from build123d import *

# Parameters (mm, degrees)
SKETCH011_W     = 266
SKETCH011_H     = 55
PAD008_DEPTH    = 4
SKETCH021_W     = 40
SKETCH021_H     = 30
POCKET004_DEPTH = 4.001
SKETCH037_R     = 3.3
HOLE002_DEPTH   = 25


with BuildPart() as part:
    # Sketch011 (on DatumPlane) → Pad008 (new body)
    with BuildSketch(Plane(origin=(0, -83, -4), x_dir=(-1, 0, 0), z_dir=(0, 1, 0))):
        with Locations((0, 23.5)):
            Rectangle(SKETCH011_W, SKETCH011_H)
    extrude(amount=PAD008_DEPTH)

    # Sketch021 (on Face5 of Pad008) → Pocket004 (cut, through all)
    with BuildSketch(Plane(origin=(0, -83, -4), x_dir=(-1, 0, 0), z_dir=(0, -1, 0))):
        with Locations((-40, 11)):
            Rectangle(SKETCH021_W, SKETCH021_H)
        with Locations((40, 11)):
            Rectangle(SKETCH021_W, SKETCH021_H)
        Polygon((100, 26), (145, 26), (145, 0.5), (155, 0.5), (155, -19.5), (125, -19.5), (125, -4), (100, -4), align=None)
        Polygon((-145, 26), (-100, 26), (-100, -4), (-125, -4), (-125, -19.5), (-155, -19.5), (-155, 0.5), (-145, 0.5), align=None)
        Polygon((-125, -47), (-100, -47), (-100, -77), (-145, -77), (-145, -51.5), (-155, -51.5), (-155, -31.5), (-125, -31.5), align=None)
        with Locations((-40, -62)):
            Rectangle(SKETCH021_W, SKETCH021_H)
        with Locations((40, -62)):
            Rectangle(SKETCH021_W, SKETCH021_H)
        Polygon((100, -47), (125, -47), (125, -31.5), (155, -31.5), (155, -51.5), (145, -51.5), (145, -77), (100, -77), align=None)
    extrude(amount=-POCKET004_DEPTH, mode=Mode.SUBTRACT)

    # Sketch037 (on Face2 of Pocket004) → Hole002 (cut)
    with BuildSketch(Plane(origin=(0, -83, -4), x_dir=(-1, 0, 0), z_dir=(0, -1, 0))):
        with Locations((-39.5, -31)):
            Circle(SKETCH037_R)
    extrude(amount=-HOLE002_DEPTH, mode=Mode.SUBTRACT)


solid = part.part
For this review, take the finished solid that the model builds, in its own axes (mm). Coordinates: 2 decimals unless noted, no trailing zeros. Loops run counter-clockwise (first coordinate to the right, second up) from the corner with the lowest first, then second, coordinate; pieces in that order, holes last. Notation, with made-up numbers: (-19.75, -36) - (32.25, -36) arc R3 ccw to (32.25, -31) - close; hole circle Ø5 at (-35.5, -36.75). An arc over 180 degrees is marked (long way). Use a Markdown table: item, result. Add a question column.
Item 1: We need section A-A (x = 39.5). Give the boundary of the cut face in (y, z), and give its area (3 significant figures).
Item 2: For line 1 (X direction, y = -80.5, z = 44.5); line 2 (Z direction, x = 39.5, y = -81.15); line 3 (X direction, y = -80.4, z = 27), list the stretches that pass through material, from the lowest coordinate up.
Item 3: We need section C-C (x = -110). Give the boundary of the cut face in (y, z).
Item 4: We need section B-B (z = 13). Give the boundary of the cut face in (x, y), and give its area (3 significant figures).
Item 5: Insertion check: pin 1 Ø2 at (x, y) = (-110, -80.5) entering from -Z; pin 2 Ø2 at (y, z) = (-81.5, 13) entering from -X; pin 3 Ø1.2 at (y, z) = (-80.5, 35) entering from +X. Each pin has a flat end and moves straight along its axis. Give the tip position at first contact, or say it passes through.
Results list:
| question | item | result |
|---|---|---|
| 1 | outline | (-83, 0) - (-79, 0) - (-79, 23.7) - (-83, 23.7) - close; (-83, 30.3) - (-79, 30.3) - (-79, 43) - (-83, 43) - close |
| 1 | area | 146 mm^2 |
| 2 | line 1 | x = -100 to -60, -20 to 20, 60 to 100 |
| 2 | line 2 | z = 0 to 23.7, 30.3 to 43 |
| 2 | line 3 | x = -133 to 36.2, 42.8 to 133 |
| 3 | outline | (-83, 0) - (-79, 0) - (-79, 43) - (-83, 43) - close |
| 4 | outline | (-125, -83) - (125, -83) - (125, -79) - (-125, -79) - close |
| 4 | area | 1,000 mm^2 |
| 5 | pin 1 | stops at z = 0 |
| 5 | pin 2 | stops at x = -125 |
| 5 | pin 3 | stops at x = 125 |
